Geometry: final body of the model. Coordinates: model frame, mm. Face numbers are marked on the shaded views. A direction names the side the tool comes from. Coordinates: 2 decimals unless noted, no trailing zeros. Order: outer loops, then holes, each group sorted by start corner. A loop starts at its lowest first (then second) coordinate and runs counter-clockwise, first axis right, second up. Notation, with made-up numbers: (-9.5, -19.5) -> (24.5, -19.5) arc R14 cw to (24.5, -15.5) -> close; hole circle Ø9 at (49.25, 76). An arc over 180 degrees is marked (long way). Use one line per item in the form item = value.
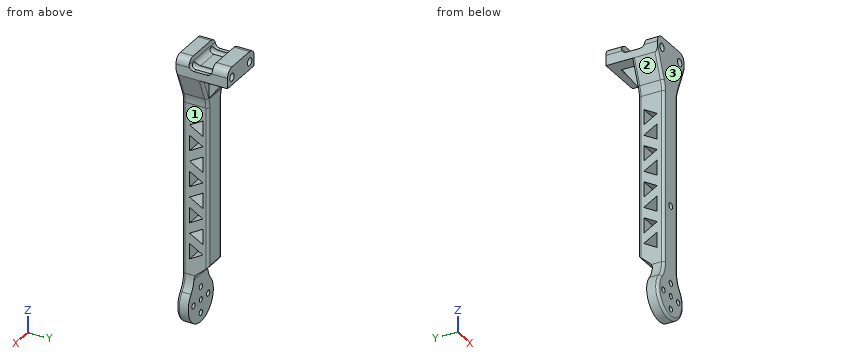
```python
from build123d import *

# Parameters (mm, degrees)
BOSS_EXTRUDE1_DEPTH     = 10
CUT_EXTRUDE1_DEPTH      = 19.370764901
CUT_EXTRUDE1_DEPTH_BACK = 1
SKETCH3_R               = 1
SKETCH3_R_2             = 1.1
CUT_EXTRUDE2_DEPTH      = 6.5
CUT_EXTRUDE2_DEPTH_BACK = 5.5000001
BOSS_EXTRUDE2_DEPTH     = 10
SKETCH5_R               = 1.5
CUT_EXTRUDE3_DEPTH      = 21.0000001
CUT_EXTRUDE4_DEPTH      = 19
CUT_EXTRUDE5_DEPTH      = 14.5000001
BOSS_EXTRUDE3_START     = -5
BOSS_EXTRUDE3_DEPTH     = 8
FILLET2_R               = 1
FILLET3_R               = 1
SKETCH11_R              = 1.25
CUT_EXTRUDE12_DEPTH     = 4


with BuildPart() as part:
    # Sketch1 → Boss-Extrude1 (new body)
    with BuildSketch(Plane(origin=(0, 0, 0), x_dir=(1, 0, 0), z_dir=(0, 1, 0))):
        with BuildLine():
            Line((3.370764901, 0), (15.370764901, 0))
            ThreePointArc((15.370764901, 0), (17.492085245, 0.878679656), (18.370764901, 3))
            Line((18.370764901, 3), (18.370764901, 7))
            Line((18.370764901, 7), (14.631969576, 16.026250381))
            ThreePointArc((14.631969576, 16.026250381), (14.062912097, 17.902181484), (13.870764901, 19.853084704))
            Line((13.870764901, 19.853084704), (13.870764901, 86.161977258))
            ThreePointArc((13.870764901, 86.161977258), (14.426762085, 89.449957004), (16.032927063, 92.372315254))
            ThreePointArc((16.032927063, 92.372315254), (9.370764901, 106.151102551), (2.708602739, 92.372315254))
            ThreePointArc((2.708602739, 92.372315254), (4.314767717, 89.449957004), (4.870764901, 86.161977258))
            Line((4.870764901, 86.161977258), (4.870764901, 19.853084704))
            ThreePointArc((4.870764901, 19.853084704), (4.678617705, 17.902181484), (4.109560226, 16.026250381))
            Line((4.109560226, 16.026250381), (0.370764901, 7))
            Line((0.370764901, 7), (0.370764901, 3))
            ThreePointArc((0.370764901, 3), (1.249444558, 0.878679656), (3.370764901, 0))
        make_face()
    extrude(amount=BOSS_EXTRUDE1_DEPTH)

    # Sketch2 → Cut-Extrude1 (cut, two sides)
    with BuildSketch(Plane(origin=(0, 0, 0), x_dir=(0, 0, -1), z_dir=(1, 0, 0))) as cut_extrude1_sk:
        with BuildLine():
            Line((79.695640218, 12.044389059), (85.546639403, 5.500402589))
            ThreePointArc((85.546639403, 5.500402589), (86.558076021, 4.761497468), (87.783067402, 4.5))
            Line((87.783067402, 4.5), (106.151102551, 4.5))
            Line((106.151102551, 4.5), (106.151102551, 14.134482691))
            Line((106.151102551, 14.134482691), (79.695640218, 14.134482691))
            Line((79.695640218, 14.134482691), (79.695640218, 12.044389059))
        make_face()
    extrude(amount=CUT_EXTRUDE1_DEPTH, mode=Mode.SUBTRACT)
    extrude(cut_extrude1_sk.sketch, amount=-CUT_EXTRUDE1_DEPTH_BACK, mode=Mode.SUBTRACT)

    # Sketch3 → Cut-Extrude2 (cut, two sides)
    with BuildSketch(Plane(origin=(0, 4.5, 0), x_dir=(1, 0, 0), z_dir=(0, 1, 0))) as cut_extrude2_sk:
        with Locations((9.370764901, 97.651102551)):
            Circle(SKETCH3_R)
        with Locations((9.370764901, 102.651102551)):
            Circle(SKETCH3_R_2)
        with Locations((14.370764901, 97.651102551)):
            Circle(SKETCH3_R_2)
        with Locations((9.370764901, 92.651102551)):
            Circle(SKETCH3_R_2)
        with Locations((4.370764901, 97.651102551)):
            Circle(SKETCH3_R_2)
    extrude(amount=CUT_EXTRUDE2_DEPTH, mode=Mode.SUBTRACT)
    extrude(cut_extrude2_sk.sketch, amount=-CUT_EXTRUDE2_DEPTH_BACK, mode=Mode.SUBTRACT)

    # Sketch4 → Boss-Extrude2 (add)
    with BuildSketch(Plane(origin=(0, 10, 0), x_dir=(1, 0, 0), z_dir=(0, 1, 0))):
        with BuildLine():
            Line((18.370764901, 7), (0.370764901, 7))
            Line((0.370764901, 7), (0.370764901, 3))
            ThreePointArc((0.370764901, 3), (1.249444558, 0.878679656), (3.370764901, 0))
            Line((3.370764901, 0), (15.370764901, 0))
            ThreePointArc((15.370764901, 0), (17.492085245, 0.878679656), (18.370764901, 3))
            Line((18.370764901, 3), (18.370764901, 7))
        make_face()
    extrude(amount=BOSS_EXTRUDE2_DEPTH)

    # Sketch5 → Cut-Extrude3 (cut, through all)
    with BuildSketch(Plane(origin=(0, 20, 0), x_dir=(1, 0, 0), z_dir=(0, 1, 0))):
        with Locations((3.370764901, 4)):
            Circle(SKETCH5_R)
        with Locations((15.370764901, 4)):
            Circle(SKETCH5_R)
    extrude(amount=-CUT_EXTRUDE3_DEPTH, mode=Mode.SUBTRACT)

    # Sketch6 → Cut-Extrude4 (cut, through all)
    with BuildSketch(Plane(origin=(18.370764901, 0, 0), x_dir=(0, 0, -1), z_dir=(1, 0, 0))):
        with BuildLine():
            Line((0, 14), (2, 14))
            ThreePointArc((2, 14), (3.414213562, 13.414213562), (4, 12))
            Line((4, 12), (4, 7))
            ThreePointArc((4, 7), (3.414213562, 5.585786438), (2, 5))
            Line((2, 5), (0, 5))
            Line((0, 5), (0, 14))
        make_face()
    extrude(amount=-CUT_EXTRUDE4_DEPTH, mode=Mode.SUBTRACT)

    # Sketch7 → Cut-Extrude5 (cut, through all)
    with BuildSketch(Plane.ZY.offset(-4.870764901)):
        Polygon((-77.173535, 7.896152423), (-80.173535, 2.7), (-74.173535, 2.7), align=None)
        Polygon((-73.173535, 7.9), (-70.173535, 2.703847577), (-67.173535, 7.9), align=None)
        Polygon((-63.173535, 7.896152423), (-66.173535, 2.7), (-60.173535, 2.7), align=None)
        Polygon((-59.173535, 7.9), (-56.173535, 2.703847577), (-53.173535, 7.9), align=None)
        Polygon((-49.173535, 7.896152423), (-52.173535, 2.7), (-46.173535, 2.7), align=None)
        Polygon((-45.173535, 7.9), (-42.173535, 2.703847577), (-39.173535, 7.9), align=None)
        Polygon((-35.173535, 7.896152423), (-38.173535, 2.7), (-32.173535, 2.7), align=None)
        Polygon((-31.173535, 7.9), (-28.173535, 2.703847577), (-25.173535, 7.9), align=None)
    extrude(amount=-CUT_EXTRUDE5_DEPTH, mode=Mode.SUBTRACT)

    # Sketch9 → Boss-Extrude3 (add)
    with BuildSketch(Plane.ZY.offset(-0.370764901).offset(BOSS_EXTRUDE3_START)):
        Polygon((-7, 16.671459489), (-7, 10), (-16.026250381, 10), align=None)
    extrude(amount=-BOSS_EXTRUDE3_DEPTH)

    # Fillet2
    fillet2_edges = [part.edges().sort_by_distance(p)[0] for p in [
        (16.501367239, 0, -11.51312519),
        (2.240162564, 0, -11.51312519),
        (4.678617705, 0, -17.902181484),
        (4.870764901, 0, -53.007530981),
        (4.314767717, 0, -89.449957004),
        (9.370764901, 0, -106.151102551),
        (14.426762085, 0, -89.449957004),
        (13.870764901, 0, -53.007530981),
        (14.062912097, 0, -17.902181484),
        (4.678617705, 10, -17.902181484),
        (2.240162564, 10, -11.51312519),
        (4.870764901, 10, -50.688309852),
        (9.370764901, 10, -81.523535),
        (14.062912097, 10, -17.902181484),
        (16.501367239, 10, -11.51312519),
        (13.870764901, 10, -50.688309852),
    ]]
    fillet(fillet2_edges, radius=FILLET2_R)

    # Fillet3
    fillet3_edges = [part.edges().sort_by_distance(p)[0] for p in [
        (9.370764901, 10, -16.026250381),
        (9.370764901, 16.671459489, -7),
    ]]
    fillet(fillet3_edges, radius=FILLET3_R)

    # Sketch11 → Cut-Extrude12 (cut)
    with BuildSketch(Plane.XZ):
        with Locations((9.370764901, -62.644330493)):
            Circle(SKETCH11_R)
    extrude(amount=-CUT_EXTRUDE12_DEPTH, mode=Mode.SUBTRACT)


solid = part.part
```
1) Section A-A, the plane z = -55. Output: boundary loops of the cut face in (x, y).
Results found:
outline = (4.87, 1) arc R1 ccw to (5.87, 0) -> (12.87, 0) arc R1 ccw to (13.87, 1) -> (13.87, 4.74) -> (4.87, 4.74) -> close; (4.87, 7.9) -> (13.87, 7.9) -> (13.87, 9) arc R1 ccw to (12.87, 10) -> (5.87, 10) arc R1 ccw to (4.87, 9) -> close
2) Material intervals for probe 1 along X at (y, z) = (14.5, -4); probe 2 along Z at (x, y) = (10.75, 17); probe 3 along Y at (x, z) = (8.5, -35), sorted ascending. Write a range as from..to.
Results found:
probe_1 = 0.37..1.87, 4.87..13.87, 16.87..18.37
probe_2 = -7.02..0
probe_3 = 0..2.7, 7.6..10
3) Access query for the marked faces 1, 2 and 3. Directions: +Z, -Z, +X, -X, +Y, -Y. A direction counts if a zero-diameter tool reaches every point of the face in a straight line with its end or side. Return the directions, or none.
Results found:
face_1 = +X, +Y, -Y
face_2 = -X, +Y, -Y
face_3 = +Z, -Z, +X, -X, -Y
4) Contact query for flat-ended pins moving along their axis: P1, Ø5, axis at y = 9, z = -35.5, coming from the +X side; P2, Ø3, axis at x = 9.37, z = -62.64, coming from the +Y side; P3, Ø6, axis at x = 6.5, y = 10, coming from the -Z side. Output: stop coordinate, or through.
Results found:
P1 = 13.87
P2 = 10
P3 = -84.21
